```python
from build123d import *

# Parameters (mm, degrees)
AUFSATZ_LINEAR_AUSTRAGEN1_DEPTH = 8
SKIZZE3_R                       = 2.5
SCHNITT_LINEAR_AUSTRAGEN1_DEPTH = 10
SCHNITT_LINEAR_AUSTRAGEN2_REACH = 25.379
SKIZZE4_R                       = 1.7
SCHNITT_LINEAR_AUSTRAGEN3_REACH = 23.099
SKIZZE5_R                       = 1.7
SKIZZE6_R                       = 1.5
SCHNITT_LINEAR_AUSTRAGEN4_DEPTH = 5


with BuildPart() as part:
    # Skizze2 → Aufsatz-Linear austragen1 (new body)
    with BuildSketch(Plane.XY):
        Polygon((-4.2, 0), (4.2, 0), (4.2, 10), (6.2, 10), (6.2, 2), (9.2, -1), (9.2, -12), (4, -12), (4, -2), (0, -2), (-2.5, -2), (-2.5, -12), (-9.2, -12), (-9.2, -1), (-6.2, 2), (-6.2, 10), (-4.2, 10), align=None)
    extrude(amount=AUFSATZ_LINEAR_AUSTRAGEN1_DEPTH)

    # Skizze3 → Schnitt-Linear austragen1 (cut)
    with BuildSketch(Plane.ZY.offset(-9.2)):
        with Locations(Location((3, -8, 0), (0, 0, 180))):
            Circle(SKIZZE3_R)
    extrude(amount=SCHNITT_LINEAR_AUSTRAGEN1_DEPTH, mode=Mode.SUBTRACT)

    # Skizze4 → Schnitt-Linear austragen2 (cut, up to next)
    with BuildSketch(Plane.ZY.offset(9.2), mode=Mode.PRIVATE) as schnitt_linear_austragen2_sk1:
        with Locations((3, -8)):
            Circle(SKIZZE4_R)
    schnitt_linear_austragen2_tool1 = extrude(schnitt_linear_austragen2_sk1.sketch, amount=-SCHNITT_LINEAR_AUSTRAGEN2_REACH, mode=Mode.PRIVATE) & part.part
    add(schnitt_linear_austragen2_tool1.solids().sort_by_distance((-9.2, -8, 3))[0], mode=Mode.SUBTRACT)

    # Skizze5 → Schnitt-Linear austragen3 (cut, up to next)
    with BuildSketch(Plane.ZY.offset(6.2), mode=Mode.PRIVATE) as schnitt_linear_austragen3_sk1:
        with Locations(Location((3, 6, 0), (0, 0, 270))):
            Circle(SKIZZE5_R)
    schnitt_linear_austragen3_tool1 = extrude(schnitt_linear_austragen3_sk1.sketch, amount=-SCHNITT_LINEAR_AUSTRAGEN3_REACH, mode=Mode.PRIVATE) & part.part
    add(schnitt_linear_austragen3_tool1.solids().sort_by_distance((-6.2, 6, 3))[0], mode=Mode.SUBTRACT)

    # Skizze6 → Schnitt-Linear austragen4 (cut)
    with BuildSketch(Plane.ZY.offset(-4.2)):
        with Locations(Location((3, 6, 0), (0, 0, 270))):
            Circle(SKIZZE6_R)
    extrude(amount=-SCHNITT_LINEAR_AUSTRAGEN4_DEPTH, mode=Mode.SUBTRACT)


solid = part.part
```
Here's how the part is built. I have some questions about the finished solid (model axes, mm). A direction names the side the tool comes from. Give positions to 0.01 mm unless a question says otherwise; leave off trailing zeros. Order: outer loops, then holes, each group sorted by start corner. A loop starts at its lowest first (then second) coordinate and runs counter-clockwise, first axis right, second up. Notation, with made-up numbers: M -15.5,-19.5 L 8.5,-19.5 A20 cw 8.5,-1.5 Z; hole C 46,-7.5 d5. An arc over 180 degrees is marked long. Use a Markdown table: item, result. Add a question column.
1. Suppose I cut it at D-D (x = -7.25). List the corners of the cut face in (y, z) for me, and give its area (3 significant figures).
2. Suppose I cut it at C-C (y = 1.5). List the corners of the cut face in (x, z) for me, and give its area (3 significant figures).
3. For pin 1 Ø2 at (y, z) = (6, 3) entering from -X; pin 2 Ø3.5 at (y, z) = (6, 3) entering from +X; pin 3 Ø4 at (y, z) = (-8, 3) entering from +X; pin 4 Ø1.5 at (y, z) = (2.5, 2) entering from -X, each with a flat end and sliding along its axis, tell me the tip position at first contact or that it passes through.
4. If we mould it in two halves opening along Z, with no side actions, what happens to faces 5 (the flat face through (-4.2, 5, 5)), 6 (the cylindrical face through (6.64, -5.56, 3.54)), 7 (the flat face through (0, -1, 0))? For each: +Z half, -Z half, draft (parallel to the pull), parting line (faces both ways), or undercut.
5. Suppose I cut it at A-A (y = 6). List the corners of the cut face in (x, z) for me.
6. Suppose I cut it at B-B (z = 6). List the corners of the cut face in (x, y) for me.
7. On a 3-axis mill with a long thin cutter (end or side, diameter ignored), from which of +Z, -Z, +X, -X, +Y, -Y can I reach the whole of each face in a straight line? I mean faces 1 (the flat face through (-6.2, 6, 5)), 2 (the flat face through (0, 0, 4)), 3 (the flat face through (4, -6, 5)), 4 (the flat face through (6.2, 6, 5)). Say none if no direction works.
8. I need wall thicknesses on probe 1 along X at (y, z) = (5.5, 6); probe 2 along X at (y, z) = (-5.5, 5.75); probe 3 along Z at (x, y) = (7.3, -8). Which ranges of each line are inside material? Lowest first, please. Write a range as from..to.
Results list:
| question | item | result |
|---|---|---|
| 1 | outline | M -12,0 L 0.95,0 L 0.95,8 L -12,8 Z; hole C -8,3 d3.4 |
| 1 | area | 94.5 mm² |
| 2 | outline | M -6.7,0 L -4.2,0 L -4.2,8 L -6.7,8 Z; M 4.2,0 L 6.7,0 L 6.7,8 L 4.2,8 Z |
| 2 | area | 40.0 mm² |
| 3 | pin 1 | passes through |
| 3 | pin 2 | stops at x = 6.2 |
| 3 | pin 3 | stops at x = -2.5 |
| 3 | pin 4 | stops at x = -6.45 |
| 4 | face 5 | draft |
| 4 | face 6 | undercut |
| 4 | face 7 | -Z half |
| 5 | outline | M -6.2,0 L -4.2,0 L -4.2,1.3 L -6.2,1.3 Z; M -6.2,4.7 L -4.2,4.7 L -4.2,8 L -6.2,8 Z; M 4.2,0 L 6.2,0 L 6.2,1.5 L 4.2,1.5 Z; M 4.2,4.5 L 6.2,4.5 L 6.2,8 L 4.2,8 Z |
| 6 | outline | M -9.2,-12 L -2.5,-12 L -2.5,-2 L 4,-2 L 4,-12 L 9.2,-12 L 9.2,-1 L 6.2,2 L 6.2,10 L 4.2,10 L 4.2,0 L -4.2,0 L -4.2,10 L -6.2,10 L -6.2,2 L -9.2,-1 Z |
| 7 | face 1 | +Z, -Z, -X, +Y |
| 7 | face 2 | +Z, -Z, +Y |
| 7 | face 3 | +Z, -Z, -Y |
| 7 | face 4 | +Z, -Z, +X, +Y |
| 8 | probe 1 | x = -6.2..-4.2, 4.2..6.2 |
| 8 | probe 2 | x = -9.2..-2.5, 4..9.2 |
| 8 | probe 3 | z = 0..0.5, 5.5..8 |
